Geometry check sheet. Reference: drawing and pictorial views, mm from the part's lowest x, y, z. Round coordinates to 2 decimals unless told otherwise and drop trailing zeros. Loops run counter-clockwise (first coordinate to the right, second up) from the corner with the lowest first, then second, coordinate; pieces in that order, holes last. Notation, with made-up numbers: (64, 61) -> (75, 61) arc R25 cw to (75, 74) -> close; hole circle Ø2 at (23, 89). An arc over 180 degrees is marked (long way). Use one line per item in the form item = value. Start each with the question number.
(1) Sectioned sample at A-A (z = 0.3). Record the cut outline in (x, y).
(2) Material ranges on probe 1 along X at (y, z) = (21.25, 0.3); probe 2 along Y at (x, z) = (6.5, 0.45), recorded low to high. Write a range as [from, to].
(3) Sectioned sample at B-B (x = 5.5). Record the cut outline in (y, z), and give its area (3 significant figures).
(4) Go/stop test with a flat-tipped pin: pin 1 (5 mm diameter, centred on x = 2.5, y = 5, fed in from -Z). Record where the tip stops, or that it passes through.
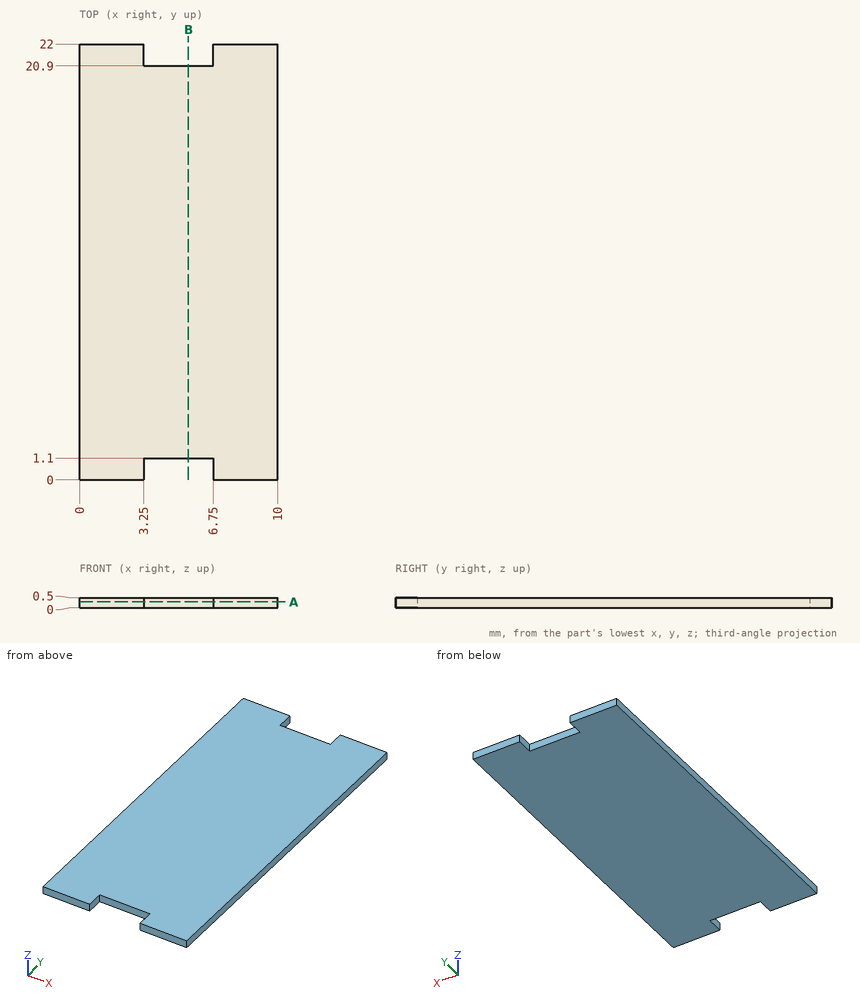
Checks:
q1.outline = (0, 0) -> (3.25, 0) -> (3.25, 1.1) -> (6.75, 1.1) -> (6.75, 0) -> (10, 0) -> (10, 22) -> (6.75, 22) -> (6.75, 20.9) -> (3.25, 20.9) -> (3.25, 22) -> (0, 22) -> close
q2.probe_1 = [0, 3.25], [6.75, 10]
q2.probe_2 = [1.1, 20.9]
q3.outline = (1.1, 0) -> (20.9, 0) -> (20.9, 0.5) -> (1.1, 0.5) -> close
q3.area = 9.90 mm2
q4.pin_1 = 0
